Can you work these out from the drawing? Everything is in mm from the part's minimum corner. Coordinates: 2 decimals unless noted, no trailing zeros. Write each loop counter-clockwise with the first axis right and the second up, starting at its lowest first coordinate (ties: lowest second). Pieces come first, ordered by that corner, then holes. Notation, with made-up numbers: M 3.5,-17 L 27.5,-17 A24 ccw 27.5,15 Z; hole C 14.5,13.25 d6. An arc over 180 degrees is marked long. Write item = value, one per line.
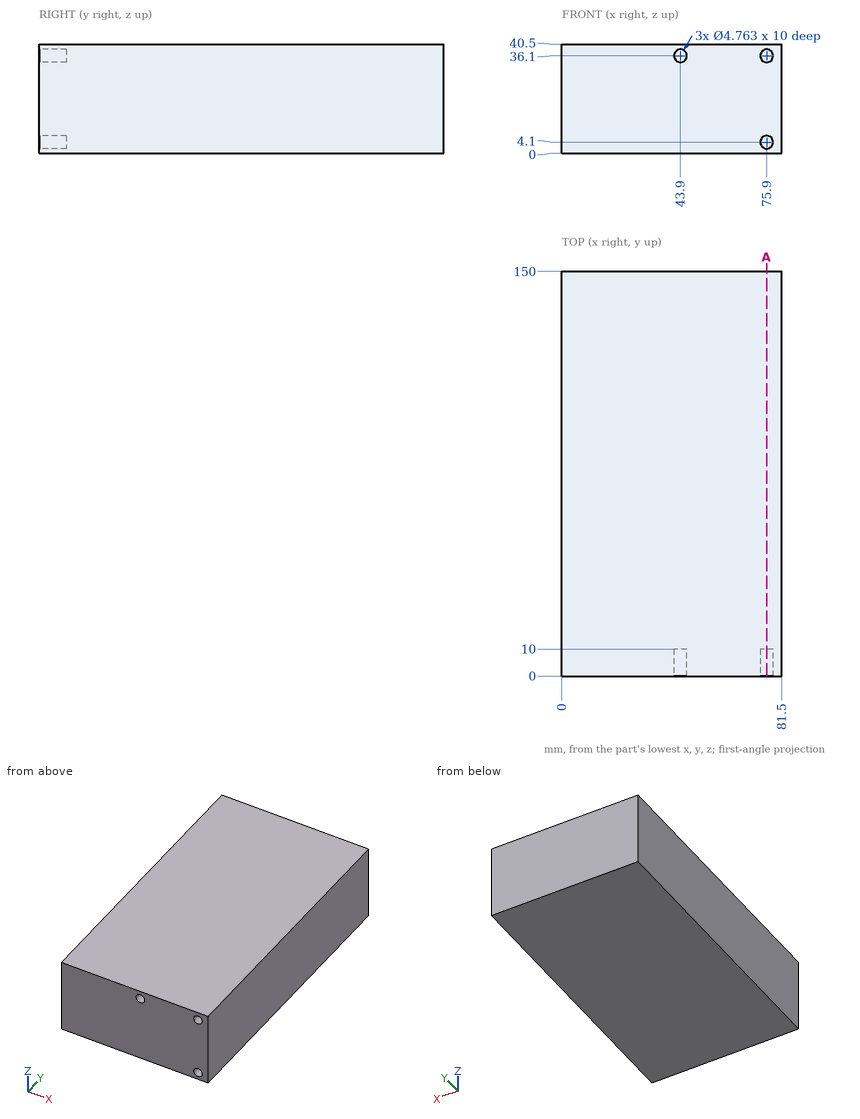
Item 1: If I drill on line 1 along Z through (x, y) = (75.9, 5); line 2 along Z through (x, y) = (43.9, 5.25); line 3 along Z through (x, y) = (43, 5) (1 decimal), over which ranges is the centre line in solid material (lowest first)?
Numbers:
line_1 = 0 to 1.72, 6.48 to 33.72, 38.48 to 40.5
line_2 = 0 to 33.72, 38.48 to 40.5
line_3 = 0 to 33.9, 38.3 to 40.5
Item 2: I'm going to push a flat-ended pin straight in: P1, Ø1.4, axis at x = 76, z = 35, coming from the -Y side. Where does the tip first touch, or does it pass through?
Numbers:
P1 = 10
Item 3: Imagine slicing it at A-A (x = 75.9). Write out the boundary of the cut face in (y, z).
Numbers:
outline = M 0,0 L 150,0 L 150,40.5 L 0,40.5 L 0,38.48 L 10,38.48 L 10,33.72 L 0,33.72 L 0,6.48 L 10,6.48 L 10,1.72 L 0,1.72 Z
